For this review, take the finished solid that the model builds, in its own axes (mm). Face numbers are marked on the shaded views. Give positions to 0.01 mm unless a question says otherwise; leave off trailing zeros. Order: outer loops, then holes, each group sorted by start corner. A loop starts at its lowest first (then second) coordinate and runs counter-clockwise, first axis right, second up. Notation, with made-up numbers: (17, 78.5) - (42, 78.5) arc R10 cw to (42, 84.5) - close; hole circle Ø2 at (74.5, 47.5). An arc over 180 degrees is marked (long way). One line per item, written item: value.
```python
from build123d import *

# Parameters (mm, degrees)
SKETCH1_R                         = 6.35
BOSS_EXTRUDE1_DEPTH               = 104.9782
M8X1_25_TAPPED_HOLE1_D            = 6.8
M8X1_25_TAPPED_HOLE1_DEPTH        = 19.7612
M8X1_25_TAPPED_HOLE1_CSINK_D      = 8.05
M8X1_25_TAPPED_HOLE1_CSINK_ANGLE  = 100
M8X1_25_TAPPED_HOLE1_TIP          = 2.042926105
F_1_4_20_TAPPED_HOLE1_D           = 5.1054
F_1_4_20_TAPPED_HOLE1_DEPTH       = 16.51
F_1_4_20_TAPPED_HOLE1_CSINK_D     = 7.62
F_1_4_20_TAPPED_HOLE1_CSINK_ANGLE = 100
F_1_4_20_TAPPED_HOLE1_TIP         = 1.533816902


with BuildPart() as part:
    # Sketch1 → Boss-Extrude1 (new body)
    with BuildSketch(Plane(origin=(0, 0, 0), x_dir=(1, 0, 0), z_dir=(0, 1, 0))):
        with Locations(Location((0, 0, 0), (0, 0, 270))):
            Circle(SKETCH1_R)
    extrude(amount=BOSS_EXTRUDE1_DEPTH)

    # M8x1.25 Tapped Hole1
    with Locations(Plane(origin=(0, 104.9782, 0), x_dir=(1, 0, 0), z_dir=(0, 1, 0))):
        with Locations((0, 0)):
            CounterSinkHole(M8X1_25_TAPPED_HOLE1_D / 2, M8X1_25_TAPPED_HOLE1_CSINK_D / 2, depth=M8X1_25_TAPPED_HOLE1_DEPTH, counter_sink_angle=M8X1_25_TAPPED_HOLE1_CSINK_ANGLE)
            with Locations((0, 0, -(M8X1_25_TAPPED_HOLE1_DEPTH + M8X1_25_TAPPED_HOLE1_TIP / 2))):  # 118° drill point
                Cone(0, M8X1_25_TAPPED_HOLE1_D / 2, M8X1_25_TAPPED_HOLE1_TIP, mode=Mode.SUBTRACT)

    # 1/4-20 Tapped Hole1
    with Locations(Plane(origin=(0, 0, 0), x_dir=(-1, 0, 0), z_dir=(0, -1, 0))):
        with Locations((0, 0)):
            CounterSinkHole(F_1_4_20_TAPPED_HOLE1_D / 2, F_1_4_20_TAPPED_HOLE1_CSINK_D / 2, depth=F_1_4_20_TAPPED_HOLE1_DEPTH, counter_sink_angle=F_1_4_20_TAPPED_HOLE1_CSINK_ANGLE)
            with Locations((0, 0, -(F_1_4_20_TAPPED_HOLE1_DEPTH + F_1_4_20_TAPPED_HOLE1_TIP / 2))):  # 118° drill point
                Cone(0, F_1_4_20_TAPPED_HOLE1_D / 2, F_1_4_20_TAPPED_HOLE1_TIP, mode=Mode.SUBTRACT)


solid = part.part
```
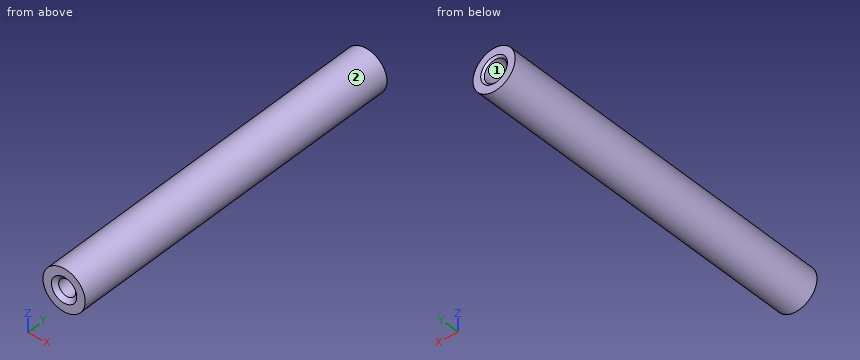
(1) For P1, Ø3, axis at x = 0, z = 0, coming from the -Y side; P2, Ø2, axis at x = -1.5, y = 22, coming from the -Z side; P3, Ø5, axis at y = 36.5, z = -4, coming from the -X side, all flat-tipped, find the tip position at first contact; note any pin that passes through.
Answers below:
P1: stops at y = 17.14
P2: stops at z = -6.33
P3: stops at x = -6.17
(2) Draft analysis for pull direction X (two halves, no side actions). For the marked faces 1 and 2, state which applies: pulls with the +X half, pulls with the -X half, needs draft (parallel to the pull), parting line crosses it, or undercut.
Answers below:
face 1: undercut
face 2: parting line crosses it
(3) Take a section at B-B (y = 67.5). Write out the cut boundary in (x, z).
Answers below:
outline: circle Ø12.7 at (0, 0)
(4) Wall thickness on line 1 (Z direction, x = 2.25, y = 6); line 2 (Z direction, x = -1, y = 10); line 3 (X direction, y = 76, z = 0.75): over which ranges is each line inside the solid? List them lowest first. Write a range as from..to.
Answers below:
line 1: z = -5.94..-1.21, 1.21..5.94
line 2: z = -6.27..-2.35, 2.35..6.27
line 3: x = -6.31..6.31
(5) Take a section at A-A (y = 12). Write out the cut boundary in (x, z).
Answers below:
outline: circle Ø12.7 at (0, 0); hole circle Ø5.11 at (0, 0)
